```python
from build123d import *

# Parameters (mm, degrees)
EXTRUDE_THIN2_DEPTH = 20.32
FILLET2_R           = 0.762


with BuildPart() as part:
    # Sketch1 → Extrude-Thin2 (new body)
    with BuildSketch(Plane.XY):
        with BuildLine():
            Line((24.32799261, 38.327319246), (24.073666549, 37.886813588))
            ThreePointArc((24.073666549, 37.886813588), (21.631585853, 35.963049129), (18.536136228, 36.250832801))
            ThreePointArc((18.536136228, 36.250832801), (0, 40.715), (-18.536136228, 36.250832801))
            ThreePointArc((-18.536136228, 36.250832801), (-21.631585853, 35.963049129), (-24.073666549, 37.886813588))
            Line((-24.073666549, 37.886813588), (-24.32799261, 38.327319246))
            ThreePointArc((-24.32799261, 38.327319246), (-24.718082956, 41.60910514), (-22.608625258, 44.153211536))
            ThreePointArc((-22.608625258, 44.153211536), (0, 49.605), (22.608625258, 44.153211536))
            ThreePointArc((22.608625258, 44.153211536), (24.718082956, 41.60910514), (24.32799261, 38.327319246))
        make_face()
        with BuildLine():
            Line((22.678214215, 39.279819246), (22.423888155, 38.839313588))
            ThreePointArc((22.423888155, 38.839313588), (21.091844139, 37.78998752), (19.403417071, 37.946960431))
            ThreePointArc((19.403417071, 37.946960431), (0, 42.62), (-19.403417071, 37.946960431))
            ThreePointArc((-19.403417071, 37.946960431), (-21.091844139, 37.78998752), (-22.423888155, 38.839313588))
            Line((-22.423888155, 38.839313588), (-22.678214215, 39.279819246))
            ThreePointArc((-22.678214215, 39.279819246), (-22.890990768, 41.069884279), (-21.740377478, 42.457578677))
            ThreePointArc((-21.740377478, 42.457578677), (0, 47.7), (21.740377478, 42.457578677))
            ThreePointArc((21.740377478, 42.457578677), (22.890990768, 41.069884279), (22.678214215, 39.279819246))
        make_face(mode=Mode.SUBTRACT)
    extrude(amount=EXTRUDE_THIN2_DEPTH)

    # Fillet2
    fillet2_edges = [part.edges().sort_by_distance(p)[0] for p in [
        (-21.091844139, 37.78998752, 0),
        (0, 42.62, 0),
        (21.091844139, 37.78998752, 0),
        (22.551051185, 39.059566417, 0),
        (22.890990768, 41.069884279, 0),
        (0, 47.7, 0),
        (-22.890990768, 41.069884279, 0),
        (-22.551051185, 39.059566417, 0),
        (-24.20082958, 38.107066417, 0),
        (-24.718082956, 41.60910514, 0),
        (0, 49.605, 0),
        (24.718082956, 41.60910514, 0),
        (24.20082958, 38.107066417, 0),
        (21.631585853, 35.963049129, 0),
        (0, 40.715, 0),
        (-21.631585853, 35.963049129, 0),
    ]]
    fillet(fillet2_edges, radius=FILLET2_R)


solid = part.part
```
The listing builds one solid part. Answer for the finished solid, in the listing's coordinates (mm). A direction names the side the tool comes from. Give positions to 0.01 mm unless a question says otherwise; leave off trailing zeros. Order: outer loops, then holes, each group sorted by start corner. A loop starts at its lowest first (then second) coordinate and runs counter-clockwise, first axis right, second up.
1) Determine the mould class of faces 1 (the face through (0.269, 40.714, 10.404)), 2 (the face through (0.11, 48.64, 0)), 3 (the face through (-0.3, 47.7, 10.4)), 4 (the face through (-24.731, 41.563, 10.404)) for opening direction X: pulls with the +X half, pulls with the -X half, needs draft (parallel to the pull), parting line crosses it, or undercut.
Reported:
face 1: undercut
face 2: needs draft
face 3: undercut
face 4: pulls with the -X half
2) Given P1, Ø5, axis at x = 9, z = 17.5, coming from the -Y side; P2, Ø5, axis at y = 46, z = 12, coming from the -X side; P3, Ø6, axis at x = 11, z = 7.5, coming from the +Y side, each flat-ended and moving along its own axis, determine where each tip first touches the part or whether it passes through.
Reported:
P1: stops at y = 39.06
P2: stops at x = -23.54
P3: stops at y = 48.96
3) Consider line 1 along Y through (x, z) = (-17, 5.75); line 2 along Y through (x, z) = (11, 6.75); line 3 along X through (y, z) = (44, 16). Determine where each line is inside the solid, lowest interval first.
Reported:
line 1: y = 37 to 39.08, 44.57 to 46.6
line 2: y = 39.2 to 41.18, 46.41 to 48.37
line 3: x = -22.88 to -18.42, 18.42 to 22.88
4) Find section A-A on z = 15. Write down the section's boundary in (x, y) (3 decimals), then the cut area to 3 significant figures.
Reported:
outline: (-24.328, 38.327) - (-24.074, 37.887) arc R4.191 ccw to (-18.536, 36.251) arc R40.715 cw to (18.536, 36.251) arc R4.191 ccw to (24.074, 37.887) - (24.328, 38.327) arc R4.191 ccw to (22.609, 44.153) arc R49.605 ccw to (-22.609, 44.153) arc R4.191 ccw to start; hole (-22.678, 39.28) - (-22.424, 38.839) arc R2.286 ccw to (-19.403, 37.947) arc R42.62 cw to (19.403, 37.947) arc R2.286 ccw to (22.424, 38.839) - (22.678, 39.28) arc R2.286 ccw to (21.74, 42.458) arc R47.7 ccw to (-21.74, 42.458) arc R2.286 ccw to start
area: 203 mm2
5) For faces 5 (the face through (22.884, 41.095, 10.404)), 6 (the face through (24.704, 41.655, 10.404)), determine the directions among +Z, -Z, +X, -X, +Y, -Y from which every point of the face is accessible in a straight line to the end or side of a thin tool.
Reported:
face 5: +Z, -Z
face 6: +Z, -Z, +X
